The model under review builds one solid part; all positions refer to its coordinate system, in mm. A direction names the side the tool comes from. Coordinates: 2 decimals unless noted, no trailing zeros. Write each loop counter-clockwise with the first axis right and the second up, starting at its lowest first coordinate (ties: lowest second). Pieces come first, ordered by that corner, then holes. Notation, with made-up numbers: (-29.5, 3.5) - (-20.5, 3.5) arc R30 cw to (-20.5, 34.5) - close; hole circle Ø4 at (-19.75, 37.5). An arc over 180 degrees is marked (long way). Put each result on its own line as item: value. Start each with the question number.
Item 1: Consider section C-C on z = 35. Give the boundary of the cut face in (x, y).
Item 2: Consider section A-A on x = -57. Give the boundary of the cut face in (y, z), then the cut area to 3 significant figures.
Item 3: Consider section B-B on y = -10.5. Give the boundary of the cut face in (x, z).
Item 4: To check wall thickness, follow L1, parallel to Z at x = -63.5, y = -3; L2, parallel to Y at x = -61.5, z = 23; L3, parallel to X at y = -13.5, z = 41. State the ranges of each line that lie inside material, in increasing order. Write a range as [from, to].
Item 5: Consider section D-D on x = -42.5. Give the boundary of the cut face in (y, z).
Item 6: For pin 1 (9.5 mm diameter, centred on x = -42, z = 22.5, fed in from +Y); pin 2 (1 mm diameter, centred on y = -13.5, z = 41, fed in from +X); pin 3 (8 mm diameter, centred on y = -7, z = 33, fed in from +X), all flat-tipped, find the tip position at first contact; note any pin that passes through.
Item 7: Machinability: for faces 1 (the face through (-53, -31.75, 25)), 2 (the face through (-56, -9, 31.57)), which of the approach directions +Z, -Z, +X, -X, +Y, -Y give a long, thin tool a straight path to every point of the face, cutting with its end or side? Answer none if there is none.
```python
from build123d import *

# Parameters (mm, degrees)
F1_DEPTH = 31.75
F3_DEPTH = 31.75
F4_W     = 19.05
F4_H     = 19.05
F5_DEPTH = 50.8


with BuildPart() as f1:
    # F0 (on Front) → F1 (new body)
    with BuildSketch(Plane.XZ):
        Polygon((-70.190806, 44.267751), (-70.190806, 12.520112), (-25.353641, 12.520112), (-25.740806, 44.267751), align=None)
    extrude(amount=F1_DEPTH)

    # F2 (on face) → F3 (cut)
    with BuildSketch(Plane.XZ.offset(31.75)):
        Polygon((-25.740806, 44.267751), (-51.140806, 44.267751), (-25.353641, 12.520112), align=None)
    extrude(amount=-F3_DEPTH, mode=Mode.SUBTRACT)

    # F4 (on face) → F5 (cut)
    with BuildSketch(Plane(origin=(-70.190806, 0, 0), x_dir=(0, -1, 0), z_dir=(-1, 0, 0))):
        with Locations((9.525, 22.045112)):
            Rectangle(F4_W, F4_H)
    extrude(amount=-F5_DEPTH, mode=Mode.SUBTRACT)


solid = f1.part
```
Report:
1. outline: (-70.19, -31.75) - (-43.61, -31.75) - (-43.61, 0) - (-70.19, 0) - close
2. outline: (-31.75, 12.52) - (-19.05, 12.52) - (-19.05, 31.57) - (0, 31.57) - (0, 44.27) - (-31.75, 44.27) - close
2. area: 645 mm²
3. outline: (-70.19, 31.57) - (-40.83, 31.57) - (-51.14, 44.27) - (-70.19, 44.27) - close
4. L1: [31.57, 44.27]
4. L2: [-31.75, -19.05]
4. L3: [-70.19, -48.49]
5. outline: (-31.75, 12.52) - (-19.05, 12.52) - (-19.05, 31.57) - (0, 31.57) - (0, 33.63) - (-31.75, 33.63) - close
6. pin 1: y = -19.05
6. pin 2: x = -48.08
6. pin 3: x = -40.83
7. face 1: +Z, -Z, +X, -X, -Y
7. face 2: -Z, +X, -X, +Y
